Could you check a few things on this drawing? It's one solid part, dimensions in mm from its lowest x, y, z. Give positions to 0.01 mm unless a question says otherwise; leave off trailing zeros. Write each loop counter-clockwise with the first axis right and the second up, starting at its lowest first coordinate (ties: lowest second). Pieces come first, ordered by that corner, then holes.
1. Suppose I cut it at C-C (z = 130). Please give me the cut outline in (x, y), and give its area (3 significant figures).
2. I'm going to push a flat-ended pin straight in: pin 1 (4 mm diameter, centred on y = 4, z = 73.5, fed in from -X). Where does the tip first touch, or does it pass through?
3. Suppose I cut it at A-A (x = 130). Please give me the cut outline in (y, z).
4. Suppose I cut it at B-B (y = 5.25). Please give me the cut outline in (x, z), and give its area (3 significant figures).
5. Suppose I cut it at D-D (x = 75). Please give me the cut outline in (y, z).
6. If I drill on probe 1 along Z at (x, y) = (20, 5); probe 2 along X at (y, z) = (4.75, 19.5); probe 3 along Z at (x, y) = (75, 1.2), over which ranges is the centre line in solid material (lowest first)?
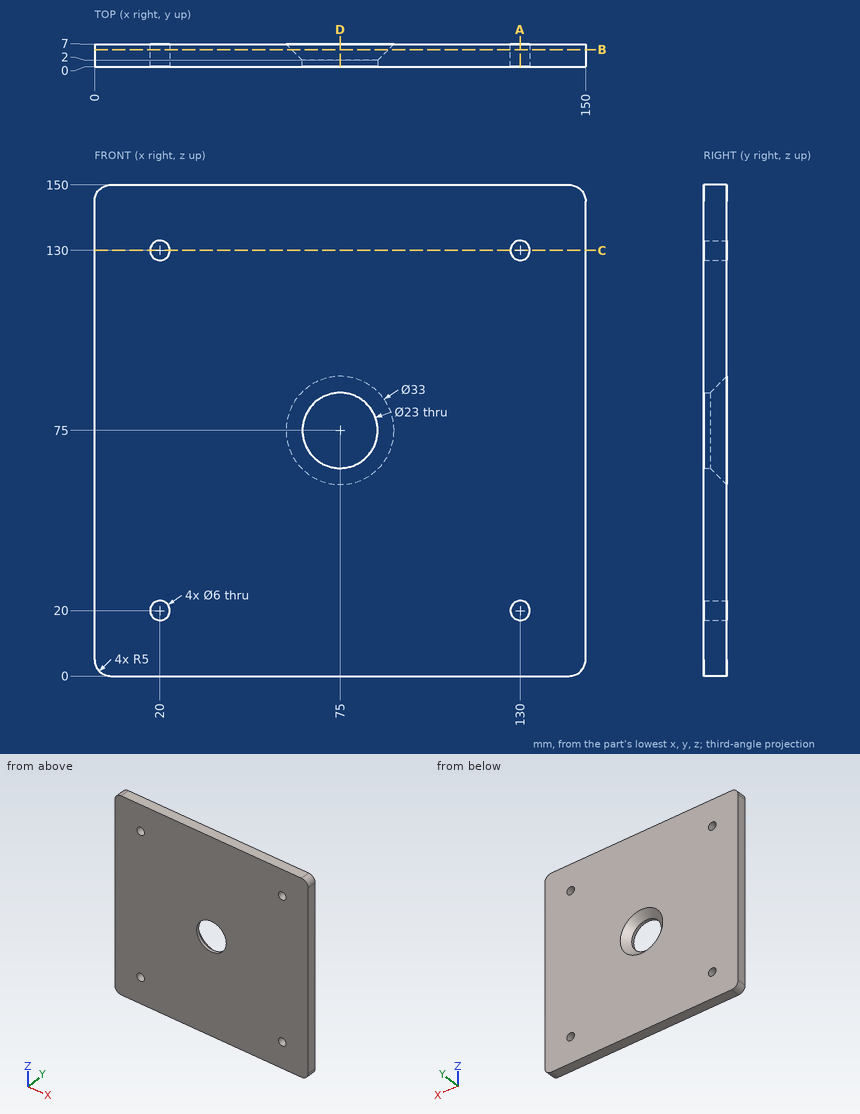
Checks:
1. outline: (0, 0) - (17, 0) - (17, 7) - (0, 7) - close; (23, 0) - (127, 0) - (127, 7) - (23, 7) - close; (133, 0) - (150, 0) - (150, 7) - (133, 7) - close
1. area: 966 mm2
2. pin 1: stops at x = 0
3. outline: (0, 0) - (7, 0) - (7, 17) - (0, 17) - close; (0, 23) - (7, 23) - (7, 127) - (0, 127) - close; (0, 133) - (7, 133) - (7, 150) - (0, 150) - close
4. outline: (0, 5) arc R5 ccw to (5, 0) - (145, 0) arc R5 ccw to (150, 5) - (150, 145) arc R5 ccw to (145, 150) - (5, 150) arc R5 ccw to (0, 145) - close; hole circle Ø6 at (20, 20); hole circle Ø6 at (20, 130); hole circle Ø29.5 at (75, 75); hole circle Ø6 at (130, 20); hole circle Ø6 at (130, 130)
4. area: 21,700 mm2
5. outline: (0, 0) - (7, 0) - (7, 58.5) - (2, 63.5) - (0, 63.5) - close; (0, 86.5) - (2, 86.5) - (7, 91.5) - (7, 150) - (0, 150) - close
6. probe 1: z = 0 to 17, 23 to 127, 133 to 150
6. probe 2: x = 0 to 17.04, 22.96 to 127.04, 132.96 to 150
6. probe 3: z = 0 to 63.5, 86.5 to 150
